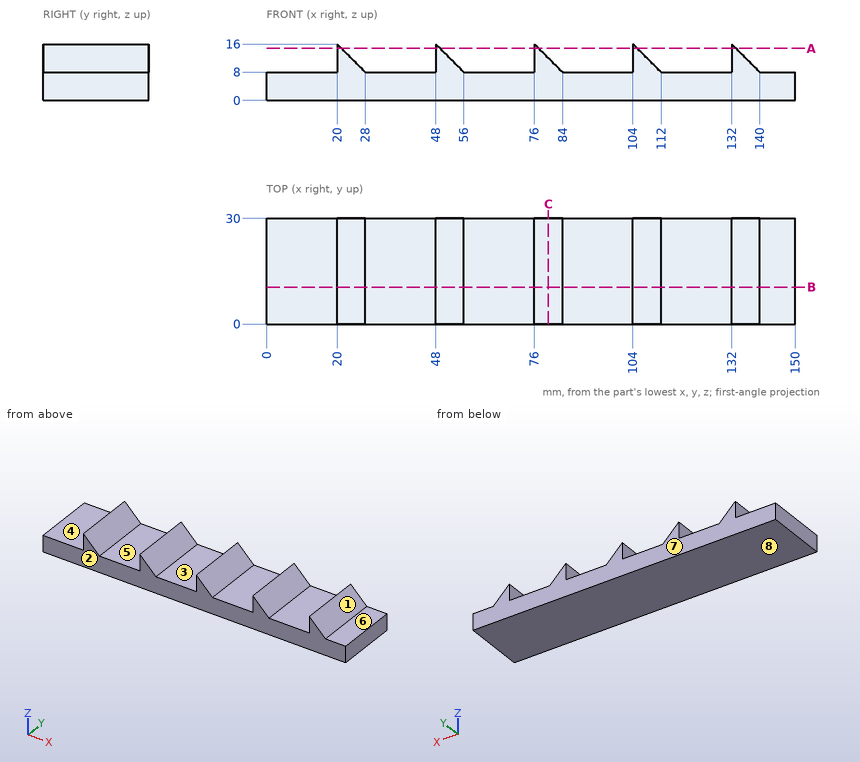
Here's the drawing with two shaded views (mm, measured from the low corner). I have some questions. A direction names the side the tool comes from. Give positions to 0.01 mm unless a question says otherwise; leave off trailing zeros. Write each loop counter-clockwise with the first axis right and the second up, starting at its lowest first coordinate (ties: lowest second). Pieces come first, ordered by that corner, then holes. Notation, with made-up numbers: (-37, -3) -> (-29, -3) arc R10 cw to (-29, 12) -> close; hole circle Ø10 at (74, 25.25). An arc over 180 degrees is marked (long way). Use one line per item in the form item = value. Start each with the question number.
1. Thinking about a two-plate mould opening in X: for the marked faces 1, 2 and 3, which applies, +X half, -X half, draft (parallel to the pull), parting line (faces both ways), or undercut?
2. On a 3-axis mill with a long thin cutter (end or side, diameter ignored), from which of +Z, -Z, +X, -X, +Y, -Y can I reach the whole of each face in a straight line? I mean the marked faces 4, 5, 6, 7 and 8. Say none if no direction works.
3. If I drill on L1, parallel to X at y = 2.75, z = 15; L2, parallel to X at y = 25.25, z = 14.75; L3, parallel to Z at x = 38, y = 27.5, over which ranges is the centre line in solid material (lowest first)?
4. Imagine slicing it at A-A on z = 14.75. List the corners of the cut face in (x, y) for me, plus the area to 4 significant figures.
5. Imagine slicing it at C-C on x = 80. List the corners of the cut face in (y, z) for me, plus the area to 3 significant figures.
6. Will these pins go through, and if not, where does the flat tip stop? pin 1 Ø11 at (x, y) = (145, 14) entering from +Z; pin 2 Ø6 at (x, y) = (14.5, 21.5) entering from +Z; pin 3 Ø4 at (x, y) = (49.5, 17) entering from -Z; pin 4 Ø4 at (y, z) = (12, 12) entering from -X.
7. Imagine slicing it at B-B on y = 10.5. List the corners of the cut face in (x, z) for me.
Entries:
q1.face_1 = +X half
q1.face_2 = draft
q1.face_3 = undercut
q2.face_4 = +Z, -X, +Y, -Y
q2.face_5 = +Z, +Y, -Y
q2.face_6 = +Z, +X, +Y, -Y
q2.face_7 = +Z, -Z, +X, -X, +Y
q2.face_8 = -Z, +X, -X, +Y, -Y
q3.L1 = 20 to 21, 48 to 49, 76 to 77, 104 to 105, 132 to 133
q3.L2 = 20 to 21.25, 48 to 49.25, 76 to 77.25, 104 to 105.25, 132 to 133.25
q3.L3 = 0 to 8
q4.outline = (20, 0) -> (21.25, 0) -> (21.25, 30) -> (20, 30) -> close; (48, 0) -> (49.25, 0) -> (49.25, 30) -> (48, 30) -> close; (76, 0) -> (77.25, 0) -> (77.25, 30) -> (76, 30) -> close; (104, 0) -> (105.25, 0) -> (105.25, 30) -> (104, 30) -> close; (132, 0) -> (133.25, 0) -> (133.25, 30) -> (132, 30) -> close
q4.area = 187.5 mm²
q5.outline = (0, 0) -> (30, 0) -> (30, 12) -> (0, 12) -> close
q5.area = 360 mm²
q6.pin_1 = 8.5
q6.pin_2 = 8
q6.pin_3 = 0
q6.pin_4 = 20
q7.outline = (0, 0) -> (150, 0) -> (150, 8) -> (140, 8) -> (132, 16) -> (132, 8) -> (112, 8) -> (104, 16) -> (104, 8) -> (84, 8) -> (76, 16) -> (76, 8) -> (56, 8) -> (48, 16) -> (48, 8) -> (28, 8) -> (20, 16) -> (20, 8) -> (0, 8) -> close
